Autodesk Inventor part; units mm, degrees
ref_plane "YZ Plane" through (0, 0, 0) normal (1, 0, 0) x (0, 1, 0)
ref_plane "XZ Plane" through (0, 0, 0) normal (0, 1, 0) x (-1, 0, 0)
ref_plane "XY Plane" through (0, 0, 0) normal (0, 0, 1) x (1, 0, 0)
sketch "Sketch1" plane through (0, 0, 0) normal (0, 1, 0) x (-1, 0, 0)
  circle A0 centre (0, 0) radius 19.05
  dimension "d0" = 38.1
extrude "Extrusion1" add sketch "Sketch1" along normal blind 67
sketch "Sketch2" plane through (0, 0, 0) normal (0, -1, 0) x (1, 0, 0)
  circle A0 centre (0, 0) radius 11.025
  dimension "d3" = 22.05
extrude "Extrusion2" cut sketch "Sketch2" against normal blind 7
ref_plane "Work Plane1" through (0, 33.5, 0) normal (0, 1, 0) x (1, 0, 0)
ref_plane "Work Plane2" through (0, 22, 0) normal (0, -1, 0) x (1, 0, 0)
sketch "Sketch4" plane through (0, 22, 0) normal (0, -1, 0) x (1, 0, 0)
  circle A0 centre (0, 0) radius 13.97
  dimension "d7" = 27.94
sketch "Sketch5" plane through (0, 7, 0) normal (0, -1, 0) x (1, 0, 0)
  circle A0 centre (0, 0) radius 11.025
  circle A1 centre (0, 0) radius 11.025
ref_plane "Work Plane3" through (0, 2, 0) normal (0, -1, 0) x (1, 0, 0)
ref_plane "Work Plane4" through (0, 12, 0) normal (0, -1, 0) x (1, 0, 0)
sketch "Sketch8" plane through (0, 12, 0) normal (0, -1, 0) x (1, 0, 0)
  circle A0 centre (0, 0) radius 9.5
  dimension "d11" = 19
sketch "Sketch9" plane through (0, 33.5, 0) normal (0, 1, 0) x (1, 0, 0)
  circle A0 centre (0, 0) radius 13.97
  dimension "d12" = 27.94
loft "Loft1" cut profiles "Sketch5", "Sketch8", "Sketch4", "Sketch9"
mirror "Mirror1" about plane through (0, 33.5, 0) normal (0, 1, 0) of "Loft1", "Extrusion2"
sketch "Sketch10" plane through (0, 67, 0) normal (0, 1, 0) x (1, 0, 0)
  circle A0 centre (0, 0) radius 16.3911
extrude "Extrusion3" add sketch "Sketch10" against normal blind 12.7
sketch "Sketch12" plane through (0, 67, 0) normal (0, 1, 0) x (1, 0, 0)
  circle A0 centre (0, 0) radius 2.8
  line L0 (0, 0) -> (0, 2) construction
  line L1 (0, 0) -> (0, -2) construction
  line L2 (0, 2) -> (-1.9596, 2)
  line L3 (0, 2) -> (1.9596, 2)
  line L4 (0, -2) -> (-1.9596, -2)
  line L5 (0, -2) -> (1.9596, -2)
  dimension "d23" = 5.6
  dimension "d24" = 2
  dimension "d25" = 2
extrude "Extrusion4" cut sketch "Sketch12" against normal blind 10 contours A0 L5 L4 L2 L3
sketch "Sketch13" plane through (0, 0, 0) normal (0, -1, 0) x (1, 0, 0)
  circle A0 centre (0, 0) radius 13.97
  circle A1 centre (0, 0) radius 28.9364
  point P0 (13.97, 0)
extrude "Extrusion5" cut sketch "Sketch13" against normal blind 63.5 contours A0 | A1
sketch "Sketch14" plane through (0, 67, 0) normal (0, 1, 0) x (1, 0, 0)
  arc A0 (1.9596, -2) -> (1.9596, 2) centre (0, 0) ccw
  circle A1 centre (0, 0) radius 6.5686
  circle A2 centre (0, 0) radius 30.6019
extrude "Extrusion6" cut sketch "Sketch14" against normal blind 63.5
properties part number "motor fit test"
Could you check a few things on this model? Use its own coordinates, in mm. A direction names the side the tool comes from. Coordinates: 2 decimals unless noted, no trailing zeros. Order: outer loops, then holes, each group sorted by start corner. A loop starts at its lowest first (then second) coordinate and runs counter-clockwise, first axis right, second up. Notation, with made-up numbers: (63, 20) - (109, 20) arc R33 ccw to (109, 57) - close; hole circle Ø2 at (24, -3). An arc over 180 degrees is marked (long way). Answer in a Markdown table with one row per item. Add a question column.
(1) If we section it at B-B, the plane z = 0: Please give me the cut outline in (x, y), then the cut area to 3 significant figures.
(2) If we section it at C-C, the plane y = 64.9: Please give me the cut outline in (x, z), then the cut area to 3 significant figures.
(3) On a 3-axis mill with a long thin cutter (end or side, diameter ignored), from which of +Z, -Z, +X, -X, +Y, -Y can I reach the whole of each face in a straight line? I mean faces 4 (the face through (3, 63.5, 0)), 5 (the face through (0, 65, -2)). Say none if no direction works.
(4) I need wall thicknesses on L1, parallel to Z at x = 0, y = 64.75; L2, parallel to Z at x = -2, y = 65.85; L3, parallel to X at y = 65.25, z = -1.25. Which ranges of each line are inside material? Lowest first, please.
(5) If we section it at A-A, the plane x = 0: Please give me the cut outline in (y, z), then the cut area to 3 significant figures.
(6) If we section it at D-D, the plane x = -5.5: Please give me the cut outline in (y, z), then the cut area to 3 significant figures.
(7) If we mould it in two halves opening along Z, with no side actions, what happens to faces 1 (the face through (-3, 67, 0)), 2 (the face through (0, 65, 2)), 3 (the face through (-1.424, 65.274, 6.412))? For each: released by +Z, released by -Z, zero draft, split by the parting line, or undercut.
Results are:
| question | item | result |
|---|---|---|
| 1 | outline | (-6.57, 63.5) - (-2.8, 63.5) - (-2.8, 67) - (-6.57, 67) - close; (2.8, 63.5) - (6.57, 63.5) - (6.57, 67) - (2.8, 67) - close |
| 1 | area | 26.4 mm2 |
| 2 | outline | circle Ø13.14 at (0, 0); hole (-1.96, -2) - (1.96, -2) arc R2.8 ccw to (1.96, 2) - (-1.96, 2) arc R2.8 ccw to start |
| 2 | area | 115 mm2 |
| 3 | face 4 | +Z, -Z, +X, -X, -Y |
| 3 | face 5 | +Y, -Y |
| 4 | L1 | z = -6.57 to -2, 2 to 6.57 |
| 4 | L2 | z = -6.26 to -1.96, 1.96 to 6.26 |
| 4 | L3 | x = -6.45 to -2.51, 2.51 to 6.45 |
| 5 | outline | (63.5, -6.57) - (67, -6.57) - (67, -2) - (63.5, -2) - close; (63.5, 2) - (67, 2) - (67, 6.57) - (63.5, 6.57) - close |
| 5 | area | 32.0 mm2 |
| 6 | outline | (63.5, -3.59) - (67, -3.59) - (67, 3.59) - (63.5, 3.59) - close |
| 6 | area | 25.1 mm2 |
| 7 | face 1 | zero draft |
| 7 | face 2 | undercut |
| 7 | face 3 | split by the parting line |
